from build123d import *

# Parameters (mm, degrees)
F1_R     = 10.99185
F2_DEPTH = 7


with BuildPart() as f2:
    # F1 (on Top) → F2 (new body)
    with BuildSketch(Plane.XY):
        Circle(F1_R)
        with BuildLine():
            ThreePointArc((10.2314, -10.263146), (13.384424, -5.556159), (14.49185, 0))
            ThreePointArc((14.49185, 0), (13.384424, 5.556159), (10.2314, 10.263146))
            ThreePointArc((10.2314, 10.263146), (9.202438, 12.74185), (10.2314, 15.220554))
            ThreePointArc((10.2314, 15.220554), (12.472478, 18.104607), (13.921297, 21.457384))
            ThreePointArc((13.921297, 21.457384), (11.583663, 34.191885), (0, 39.97555))
            ThreePointArc((0, 39.97555), (-11.583663, 34.191885), (-13.921297, 21.457384))
            ThreePointArc((-13.921297, 21.457384), (-12.472478, 18.104607), (-10.2314, 15.220554))
            ThreePointArc((-10.2314, 15.220554), (-9.202438, 12.74185), (-10.2314, 10.263146))
            ThreePointArc((-10.2314, 10.263146), (-14.49185, 0), (-10.2314, -10.263146))
            ThreePointArc((-10.2314, -10.263146), (-9.202438, -12.74185), (-10.2314, -15.220554))
            ThreePointArc((-10.2314, -15.220554), (-12.472478, -18.104607), (-13.921297, -21.457384))
            ThreePointArc((-13.921297, -21.457384), (-11.583663, -34.191885), (0, -39.97555))
            ThreePointArc((0, -39.97555), (11.583663, -34.191885), (13.921297, -21.457384))
            ThreePointArc((13.921297, -21.457384), (12.472478, -18.104607), (10.2314, -15.220554))
            ThreePointArc((10.2314, -15.220554), (9.202438, -12.74185), (10.2314, -10.263146))
        make_face()
        with Locations((0, -25.4837)):
            Circle(F1_R, mode=Mode.SUBTRACT)
        Circle(F1_R, mode=Mode.SUBTRACT)
        with Locations((0, 25.4837)):
            Circle(F1_R, mode=Mode.SUBTRACT)
        with BuildLine():
            Line((25.880013, -21.519277), (13.921297, -21.457384))
            ThreePointArc((13.921297, -21.457384), (11.583663, -34.191885), (0, -39.97555))
            ThreePointArc((0, -39.97555), (15.893466, -34.888855), (25.880013, -21.519277))
        make_face()
        with BuildLine():
            ThreePointArc((0, 39.97555), (11.583663, 34.191885), (13.921297, 21.457384))
            Line((13.921297, 21.457384), (25.880013, 21.519277))
            ThreePointArc((25.880013, 21.519277), (15.893466, 34.888855), (0, 39.97555))
        make_face()
        with BuildLine():
            ThreePointArc((-25.880013, -21.519277), (-15.893466, -34.888855), (0, -39.97555))
            ThreePointArc((0, -39.97555), (-11.583663, -34.191885), (-13.921297, -21.457384))
            Line((-13.921297, -21.457384), (-25.880013, -21.519277))
        make_face()
        with BuildLine():
            ThreePointArc((-13.921297, 21.457384), (-11.583663, 34.191885), (0, 39.97555))
            ThreePointArc((0, 39.97555), (-15.893466, 34.888855), (-25.880013, 21.519277))
            Line((-25.880013, 21.519277), (-13.921297, 21.457384))
        make_face()
    extrude(amount=F2_DEPTH)


solid = f2.part
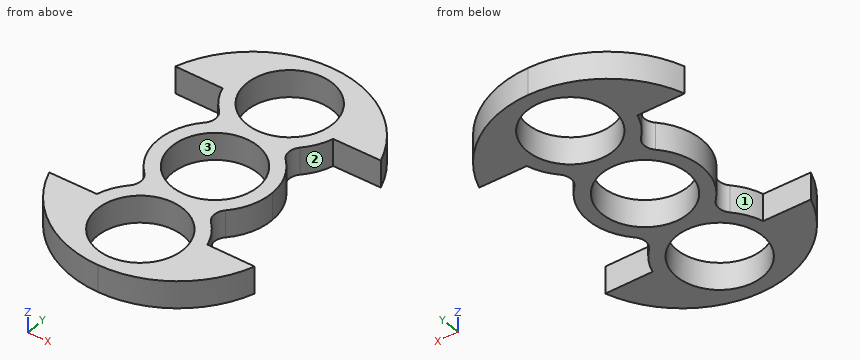
Geometry check sheet. Reference: the model listing, model coordinates, mm. Face numbers are marked on the shaded views. Round coordinates to 2 decimals unless told otherwise and drop trailing zeros. Write each loop counter-clockwise with the first axis right and the second up, starting at its lowest first coordinate (ties: lowest second). Pieces come first, ordered by that corner, then holes.
Item 1: Go/stop test with flat-tipped pins: pin 1 Ø13 at (x, y) = (0, 25.48) entering from +Z; pin 2 Ø1.5 at (x, z) = (10.5, 6) entering from +Y; pin 3 Ø2 at (x, z) = (18, 2.5) entering from +Y. Record where each tip stops, or that it passes through.
Determined:
pin 1: passes through
pin 2: stops at y = 38.18
pin 3: stops at y = 34.06
Item 2: Section check D-D (z = 3.75). Record the boundary of the cut face in (x, y).
Determined:
outline: (-25.88, -21.52) arc R27.37 ccw to (0, -39.98) arc R27.37 ccw to (25.88, -21.52) - (13.92, -21.46) arc R14.49 ccw to (10.23, -15.22) arc R3.5 cw to (10.23, -10.26) arc R14.49 ccw to (14.49, 0) arc R14.49 ccw to (10.23, 10.26) arc R3.5 cw to (10.23, 15.22) arc R14.49 ccw to (13.92, 21.46) - (25.88, 21.52) arc R27.37 ccw to (0, 39.98) arc R27.37 ccw to (-25.88, 21.52) - (-13.92, 21.46) arc R14.49 ccw to (-10.23, 15.22) arc R3.5 cw to (-10.23, 10.26) arc R14.49 ccw to (-10.23, -10.26) arc R3.5 cw to (-10.23, -15.22) arc R14.49 ccw to (-13.92, -21.46) - close; hole circle Ø21.98 at (0, -25.48); hole circle Ø21.98 at (0, 0); hole circle Ø21.98 at (0, 25.48)
Item 3: Section check C-C (x = 8). Record the boundary of the cut face in (y, z).
Determined:
outline: (-38.78, 0) - (-33.02, 0) - (-33.02, 7) - (-38.78, 7) - close; (-17.95, 0) - (-7.54, 0) - (-7.54, 7) - (-17.95, 7) - close; (7.54, 0) - (17.95, 0) - (17.95, 7) - (7.54, 7) - close; (33.02, 0) - (38.78, 0) - (38.78, 7) - (33.02, 7) - close
Item 4: Section check B-B (y = 1.5). Record the boundary of the cut face in (x, z).
Determined:
outline: (-14.41, 0) - (-10.89, 0) - (-10.89, 7) - (-14.41, 7) - close; (10.89, 0) - (14.41, 0) - (14.41, 7) - (10.89, 7) - close
Item 5: Material ranges on line 1 along X through (y, z) = (-4, 0.5); line 2 along Y through (x, z) = (6, 5.5); line 3 along Y through (x, z) = (-5.5, 3.5), recorded low to high.
Determined:
line 1: x = -13.93 to -10.24, 10.24 to 13.93
line 2: y = -39.31 to -34.69, -16.27 to -9.21, 9.21 to 16.27, 34.69 to 39.31
line 3: y = -39.42 to -35, -15.97 to -9.52, 9.52 to 15.97, 35 to 39.42
Item 6: Mould release check, pull along X, two halves, no side actions. Record for the marked faces 1, 2 and 3: +X half, -X half, draft (parallel to the pull), parting line (faces both ways), or undercut.
Determined:
face 1: -X half
face 2: +X half
face 3: undercut
Item 7: Section check A-A (x = 19). Record the boundary of the cut face in (y, z).
Determined:
outline: (-32.31, 0) - (-21.48, 0) - (-21.48, 7) - (-32.31, 7) - close; (21.48, 0) - (32.31, 0) - (32.31, 7) - (21.48, 7) - close
